Answer from the drawing. Dimensions are ordinates in mm from the lowest x, y and z of the part. A direction names the side the tool comes from. Give positions to 0.01 mm unless a question says otherwise; leave off trailing zeros. Order: outer loops, then holes, each group sorted by start corner. A loop starts at its lowest first (then second) coordinate and runs counter-clockwise, first axis right, second up.
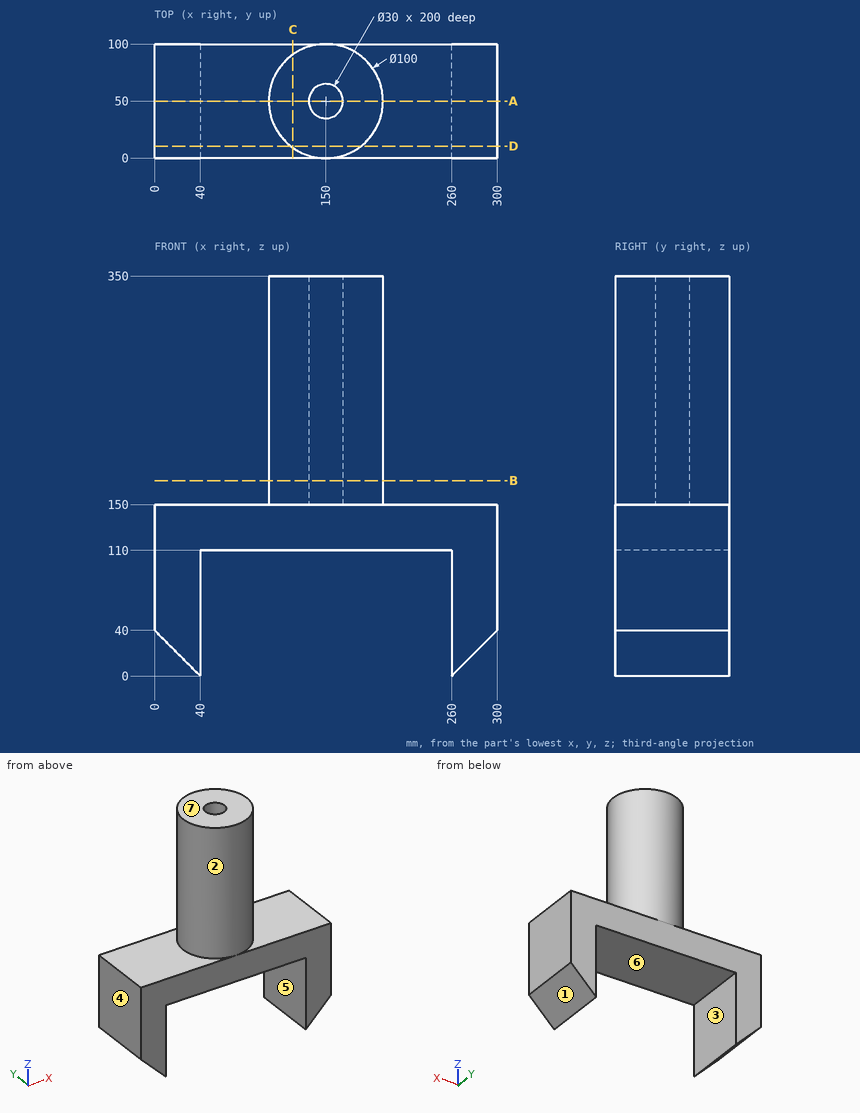
1. The part is cut by section B-B (z = 171). Write down the section's boundary in (x, y).
Findings below:
outline: circle Ø100 at (150, 50); hole circle Ø30 at (150, 50)
2. Given P1, Ø10, axis at y = 23.5, z = 224, coming from the +X side; P2, Ø1.5, axis at x = 235.5, y = 53.5, coming from the -Z side; P3, Ø8, axis at x = 70, y = 85, coming from the +Z side, each flat-ended and moving along its own axis, determine where each tip first touches the part or whether it passes through.
Findings below:
P1: stops at x = 195.14
P2: stops at z = 110
P3: stops at z = 150
3. The part is cut by section C-C (x = 121). Write down the section's boundary in (y, z).
Findings below:
outline: (0, 110) - (100, 110) - (100, 150) - (90.73, 150) - (90.73, 350) - (9.27, 350) - (9.27, 150) - (0, 150) - close
4. The part is cut by section D-D (y = 10.5). Write down the section's boundary in (x, z), then the cut area to 3 significant figures.
Findings below:
outline: (0, 40) - (40, 0) - (40, 110) - (260, 110) - (260, 0) - (300, 40) - (300, 150) - (180.66, 150) - (180.66, 350) - (119.34, 350) - (119.34, 150) - (0, 150) - close
area: 31,500 mm2
5. Straight lines are drawn through the part: probe 1 along Y at (x, z) = (150, 289); probe 2 along X at (y, z) = (95.5, 52.5); probe 3 along Y at (x, z) = (145.5, 265). For each, find the intervals that lie inside material, in ascending order.
Findings below:
probe 1: y = 0 to 35, 65 to 100
probe 2: x = 0 to 40, 260 to 300
probe 3: y = 0.2 to 35.69, 64.31 to 99.8
6. The mould has two halves that part along X. Classify the marked faces 4, 5, 6 and 7: pulls with the +X half, pulls with the -X half, needs draft (parallel to the pull), parting line crosses it, or undercut.
Findings below:
face 4: pulls with the -X half
face 5: undercut
face 6: undercut
face 7: needs draft
7. The part is cut by section A-A (y = 50). Write down the section's boundary in (x, z).
Findings below:
outline: (0, 40) - (40, 0) - (40, 110) - (260, 110) - (260, 0) - (300, 40) - (300, 150) - (200, 150) - (200, 350) - (165, 350) - (165, 150) - (135, 150) - (135, 350) - (100, 350) - (100, 150) - (0, 150) - close
8. Which of the six approach directions +Z, -Z, +X, -X, +Y, -Y give full straight-line access (tool end or side, diameter ignored) to the marked faces 1, 2 and 3?
Findings below:
face 1: -Z, +X, +Y, -Y
face 2: +Z
face 3: -Z, +Y, -Y
